from build123d import *

# Parameters (mm, degrees)
F0_R     = 42.5
F1_DEPTH = 91
F5_T     = -2.5
F6_R     = 1


with BuildPart() as f1:
    # F0 (on Top) → F1 (new body)
    with BuildSketch(Plane.XY):
        Circle(F0_R)
    extrude(amount=F1_DEPTH)

    # F5
    f5_openings = [f1.faces().sort_by_distance(p)[0] for p in [
        (0, 0, 91),
    ]]
    offset(amount=F5_T, openings=f5_openings)

    # F6
    f6_edges = [f1.edges().sort_by_distance(p)[0] for p in [
        (-40, 0, 2.5),
        (42.5, 0, 45.5),
        (-42.5, 0, 0),
        (-42.5, 0, 91),
        (40, 0, 46.75),
        (-40, 0, 91),
    ]]
    fillet(f6_edges, radius=F6_R)


solid = f1.part
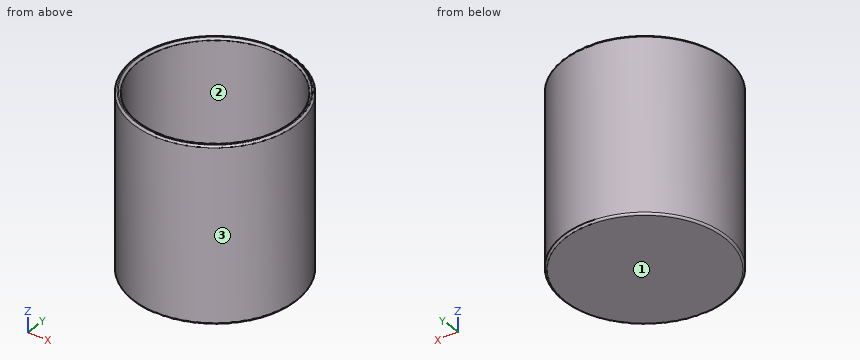
Model file for the job. Use its own axes, mm. Face numbers are marked on the shaded views. Give positions to 0.01 mm unless a question says otherwise; leave off trailing zeros. Loops run counter-clockwise (first coordinate to the right, second up) from the corner with the lowest first, then second, coordinate; pieces in that order, holes last.
1) Flat gauge pins, fed straight in: pin 1 Ø8 at (x, z) = (-22, 20.5) entering from -Y; pin 2 Ø3 at (y, z) = (-27.5, 81.5) entering from -X; pin 3 Ø2 at (x, z) = (2, 78) entering from -Y. Where does each tip first touch, or does it go through?
2) Wall check: line 1 (Y direction, x = 0, z = 32); line 2 (Z direction, x = 30.5, y = 14.5); line 3 (Y direction, x = -14.5, z = 75). Give the ranges that are in metal, low to high.
3) Pull direction X, two halves, no side cores. Call the marked faces 1, 2 and 3: +X half, -X half, draft (parallel to the pull), parting line (faces both ways), or undercut.
4) Saw through at C-C (z = 35). Write the cut outline in (x, y).
5) Saw through at A-A (x = 0). Write the cut outline in (y, z).
Answer block:
1. pin 1: stops at y = -38.5
1. pin 2: stops at x = -33.62
1. pin 3: stops at y = -42.49
2. line 1: y = -42.5 to -40, 40 to 42.5
2. line 2: z = 0 to 2.5
2. line 3: y = -39.95 to -37.28, 37.28 to 39.95
3. face 1: draft
3. face 2: undercut
3. face 3: parting line
4. outline: circle Ø85 at (0, 0); hole circle Ø80 at (0, 0)
5. outline: (-42.5, 1) arc R1 ccw to (-41.5, 0) - (41.5, 0) arc R1 ccw to (42.5, 1) - (42.5, 90) arc R1 ccw to (41.5, 91) - (41, 91) arc R1 ccw to (40, 90) - (40, 3.5) arc R1 cw to (39, 2.5) - (-39, 2.5) arc R1 cw to (-40, 3.5) - (-40, 90) arc R1 ccw to (-41, 91) - (-41.5, 91) arc R1 ccw to (-42.5, 90) - close
